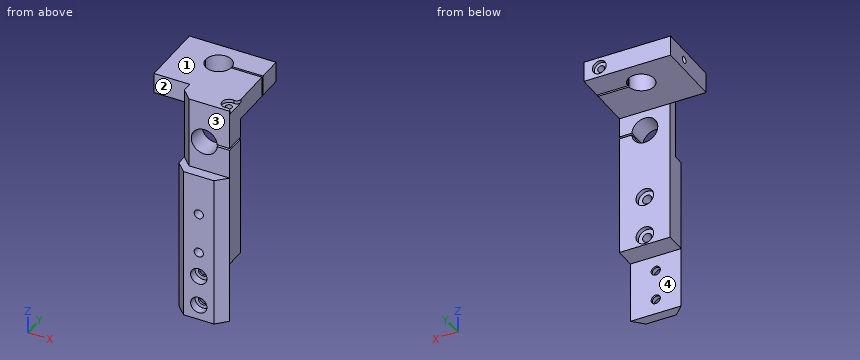
from build123d import *

# Parameters (mm, degrees)
SKETCH1_W                       = 24.85
SKETCH1_H                       = 110
BOSS_EXTRUDE1_DEPTH             = 15
SKETCH2_W                       = 24.85
SKETCH2_H                       = 30
CUT_EXTRUDE1_DEPTH              = 10
SKETCH4_W                       = 35
SKETCH4_H                       = 5
CUT_EXTRUDE3_DEPTH              = 63.189408262
SKETCH5_W                       = 17.575
SKETCH5_H                       = 10
BOSS_EXTRUDE2_DEPTH             = 10
SKETCH6_W                       = 42.425
SKETCH6_H                       = 10
BOSS_EXTRUDE3_DEPTH             = 32.42
CHAMFER2_SIZE                   = 5
SKETCH7_R                       = 6.375
CUT_EXTRUDE4_DEPTH              = 71.541168122
SKETCH8_R                       = 6.375
CUT_EXTRUDE5_DEPTH              = 115.667590888
CBORE_FOR_M4_SHCS1_D            = 4.5
CBORE_FOR_M4_SHCS1_DEPTH        = 10.1
CBORE_FOR_M4_SHCS1_CBORE_D      = 8
CBORE_FOR_M4_SHCS1_CBORE_DEPTH  = 4
CBORE_FOR_M4_SHCS1_TIP          = 1.351936393
M4X0_7_TAPPED_HOLE1_D           = 3.3
SKETCH15_W                      = 17.575
SKETCH15_H                      = 10
CUT_EXTRUDE6_DEPTH              = 115.667590888
CHAMFER6_SIZE                   = 5
SKETCH16_W                      = 15
SKETCH16_H                      = 1
CUT_EXTRUDE7_DEPTH              = 71.541168122
CBORE_FOR_M3_SBHCS1_D           = 3.2
CBORE_FOR_M3_SBHCS1_DEPTH       = 19.5
CBORE_FOR_M3_SBHCS1_CBORE_D     = 6.7
CBORE_FOR_M3_SBHCS1_CBORE_DEPTH = 1.65
M3X0_5_TAPPED_HOLE1_D           = 2.5
M3X0_5_TAPPED_HOLE1_DEPTH       = 7.5
M3X0_5_TAPPED_HOLE1_TIP         = 0.751075774
CUT_EXTRUDE8_REACH              = 125.485
SKETCH24_W                      = 22
SKETCH24_H                      = 1
CBORE_FOR_M3_SBHCS2_D           = 3.4
CBORE_FOR_M3_SBHCS2_DEPTH       = 11.92
CBORE_FOR_M3_SBHCS2_CBORE_D     = 6.7
CBORE_FOR_M3_SBHCS2_CBORE_DEPTH = 1.65
M3X0_5_TAPPED_HOLE2_D           = 2.5
M3X0_5_TAPPED_HOLE2_DEPTH       = 7.5
M3X0_5_TAPPED_HOLE2_TIP         = 0.751075774
M4X0_7_TAPPED_HOLE2_D           = 3.3
M4X0_7_TAPPED_HOLE2_DEPTH       = 10.1
M4X0_7_TAPPED_HOLE2_TIP         = 0.991420021
CBORE_FOR_M4_SBHCS1_D           = 4.5
CBORE_FOR_M4_SBHCS1_CBORE_D     = 8.6
CBORE_FOR_M4_SBHCS1_CBORE_DEPTH = 2.2
FILLET2_R                       = 2


with BuildPart() as part:
    # Sketch1 → Boss-Extrude1 (new body)
    with BuildSketch(Plane(origin=(0, 0, 0), x_dir=(1, 0, 0), z_dir=(0, 1, 0))):
        Rectangle(SKETCH1_W, SKETCH1_H)
    extrude(amount=BOSS_EXTRUDE1_DEPTH)

    # Sketch2 → Cut-Extrude1 (cut)
    with BuildSketch(Plane(origin=(0, 15, 0), x_dir=(1, 0, 0), z_dir=(0, 1, 0))):
        with Locations((0, 40)):
            Rectangle(SKETCH2_W, SKETCH2_H)
    extrude(amount=-CUT_EXTRUDE1_DEPTH, mode=Mode.SUBTRACT)

    # Sketch4 → Cut-Extrude3 (cut, through all)
    with BuildSketch(Plane.ZY.offset(12.425)):
        with Locations((37.5, 2.5)):
            Rectangle(SKETCH4_W, SKETCH4_H)
    extrude(amount=-CUT_EXTRUDE3_DEPTH, mode=Mode.SUBTRACT)

    # Sketch5 → Boss-Extrude2 (add)
    with BuildSketch(Plane(origin=(0, 15, 0), x_dir=(1, 0, 0), z_dir=(0, 1, 0))):
        with Locations((-21.2125, -50)):
            Rectangle(SKETCH5_W, SKETCH5_H)
    extrude(amount=-BOSS_EXTRUDE2_DEPTH)

    # Sketch6 → Boss-Extrude3 (add)
    with BuildSketch(Plane(origin=(0, 15, 0), x_dir=(1, 0, 0), z_dir=(0, 1, 0))):
        with Locations((-8.7875, -50)):
            Rectangle(SKETCH6_W, SKETCH6_H)
    extrude(amount=BOSS_EXTRUDE3_DEPTH)

    # Chamfer2
    chamfer2_edges = [part.edges().sort_by_distance(p)[0] for p in [
        (12.425, 0, -17.5),
        (-12.425, 0, -17.5),
    ]]
    chamfer(chamfer2_edges, length=CHAMFER2_SIZE)

    # Sketch7 → Cut-Extrude4 (cut, through all)
    with BuildSketch(Plane(origin=(0, 15, 0), x_dir=(1, 0, 0), z_dir=(0, 1, 0))):
        with Locations(Location((0, -35, 0), (0, 0, 270))):
            Circle(SKETCH7_R)
    extrude(amount=-CUT_EXTRUDE4_DEPTH, mode=Mode.SUBTRACT)

    # Sketch8 → Cut-Extrude5 (cut, through all)
    with BuildSketch(Plane(origin=(0, 0, 45), x_dir=(-1, 0, 0), z_dir=(0, 0, -1))):
        with Locations((9, 35)):
            Circle(SKETCH8_R)
    extrude(amount=-CUT_EXTRUDE5_DEPTH, mode=Mode.SUBTRACT)

    # CBORE for M4 SHCS1
    with Locations(Plane(origin=(0, 0, 0), x_dir=(-1, 0, 0), z_dir=(0, -1, 0))):
        with Locations((0, 47.5), (0, 32.5)):
            CounterBoreHole(CBORE_FOR_M4_SHCS1_D / 2, CBORE_FOR_M4_SHCS1_CBORE_D / 2, CBORE_FOR_M4_SHCS1_CBORE_DEPTH, depth=CBORE_FOR_M4_SHCS1_DEPTH)
            with Locations((0, 0, -(CBORE_FOR_M4_SHCS1_DEPTH + CBORE_FOR_M4_SHCS1_TIP / 2))):  # 118° drill point
                Cone(0, CBORE_FOR_M4_SHCS1_D / 2, CBORE_FOR_M4_SHCS1_TIP, mode=Mode.SUBTRACT)

    # M4x0.7 Tapped Hole1 (through all)
    with Locations(Plane(origin=(0, 0, 0), x_dir=(-1, 0, 0), z_dir=(0, -1, 0))):
        with Locations((0, 20), (0, 0)):
            Hole(M4X0_7_TAPPED_HOLE1_D / 2)

    # Sketch15 → Cut-Extrude6 (cut, through all)
    with BuildSketch(Plane(origin=(0, 0, 45), x_dir=(-1, 0, 0), z_dir=(0, 0, -1))):
        with Locations((21.2125, 10)):
            Rectangle(SKETCH15_W, SKETCH15_H)
    extrude(amount=-CUT_EXTRUDE6_DEPTH, mode=Mode.SUBTRACT)

    # Chamfer6
    chamfer6_edges = [part.edges().sort_by_distance(p)[0] for p in [
        (-12.425, 5, 37.5),
    ]]
    chamfer(chamfer6_edges, length=CHAMFER6_SIZE)

    # Sketch16 → Cut-Extrude7 (cut, through all)
    with BuildSketch(Plane(origin=(0, 15, 0), x_dir=(1, 0, 0), z_dir=(0, 1, 0))):
        with Locations((12.425, -35)):
            Rectangle(SKETCH16_W, SKETCH16_H)
    extrude(amount=-CUT_EXTRUDE7_DEPTH, mode=Mode.SUBTRACT)

    # CBORE for M3 SBHCS1
    with Locations(Plane(origin=(9.390180955, 10, 55), x_dir=(1, 0, 0), z_dir=(0, 0, 1))):
        with Locations((0, 0)):
            CounterBoreHole(CBORE_FOR_M3_SBHCS1_D / 2, CBORE_FOR_M3_SBHCS1_CBORE_D / 2, CBORE_FOR_M3_SBHCS1_CBORE_DEPTH, depth=CBORE_FOR_M3_SBHCS1_DEPTH)

    # M3x0.5 Tapped Hole1
    with Locations(Plane.XY.offset(34.5)):
        with Locations((9.390180955, 10)):
            Hole(M3X0_5_TAPPED_HOLE1_D / 2, depth=M3X0_5_TAPPED_HOLE1_DEPTH)
            with Locations((0, 0, -(M3X0_5_TAPPED_HOLE1_DEPTH + M3X0_5_TAPPED_HOLE1_TIP / 2))):  # 118° drill point
                Cone(0, M3X0_5_TAPPED_HOLE1_D / 2, M3X0_5_TAPPED_HOLE1_TIP, mode=Mode.SUBTRACT)

    # Sketch24 → Cut-Extrude8 (cut, up to next)
    with BuildSketch(Plane.XY.offset(55), mode=Mode.PRIVATE) as cut_extrude8_sk1:
        with Locations((1.425, 35)):
            Rectangle(SKETCH24_W, SKETCH24_H)
    cut_extrude8_tool1 = extrude(cut_extrude8_sk1.sketch, amount=-CUT_EXTRUDE8_REACH, mode=Mode.PRIVATE) & part.part
    add(cut_extrude8_tool1.solids().sort_by_distance((1.425, 35, 55))[0], mode=Mode.SUBTRACT)

    # CBORE for M3 SBHCS2
    with Locations(Plane(origin=(0, 47.42, 0), x_dir=(1, 0, 0), z_dir=(0, 1, 0))):
        with Locations((4.890180955, -50)):
            CounterBoreHole(CBORE_FOR_M3_SBHCS2_D / 2, CBORE_FOR_M3_SBHCS2_CBORE_D / 2, CBORE_FOR_M3_SBHCS2_CBORE_DEPTH, depth=CBORE_FOR_M3_SBHCS2_DEPTH)

    # M3x0.5 Tapped Hole2
    with Locations(Plane(origin=(0, 34.5, 0), x_dir=(1, 0, 0), z_dir=(0, 1, 0))):
        with Locations((4.890180955, -50)):
            Hole(M3X0_5_TAPPED_HOLE2_D / 2, depth=M3X0_5_TAPPED_HOLE2_DEPTH)
            with Locations((0, 0, -(M3X0_5_TAPPED_HOLE2_DEPTH + M3X0_5_TAPPED_HOLE2_TIP / 2))):  # 118° drill point
                Cone(0, M3X0_5_TAPPED_HOLE2_D / 2, M3X0_5_TAPPED_HOLE2_TIP, mode=Mode.SUBTRACT)

    # M4x0.7 Tapped Hole2
    with Locations(Plane.ZY.offset(30)):
        with Locations((50, 35)):
            Hole(M4X0_7_TAPPED_HOLE2_D / 2, depth=M4X0_7_TAPPED_HOLE2_DEPTH)
            with Locations((0, 0, -(M4X0_7_TAPPED_HOLE2_DEPTH + M4X0_7_TAPPED_HOLE2_TIP / 2))):  # 118° drill point
                Cone(0, M4X0_7_TAPPED_HOLE2_D / 2, M4X0_7_TAPPED_HOLE2_TIP, mode=Mode.SUBTRACT)

    # CBORE for M4 SBHCS1 (through all)
    with Locations(Plane(origin=(0, 15, 0), x_dir=(1, 0, 0), z_dir=(0, 1, 0))):
        with Locations((0, 20), (0, 0)):
            CounterBoreHole(CBORE_FOR_M4_SBHCS1_D / 2, CBORE_FOR_M4_SBHCS1_CBORE_D / 2, CBORE_FOR_M4_SBHCS1_CBORE_DEPTH)

    # Fillet2
    # the kernel refuses this fillet: 2 mm, written as the material it takes off along each edge
    with BuildSketch(Plane(origin=(12.425, 11.418581462, 53.35), x_dir=(0, 1, 0), z_dir=(0, 0, 1))) as fillet2_piece_1:
        with BuildLine():
            CenterArc((3.83038506, 2), FILLET2_R, 168.847320213, 101.152679787)
            Line((1.868154584, 2.386848241), (1.828909975, 2.394585206))
            ThreePointArc((1.828909975, 2.394585206), (1.187961295, 0.994712466), (-0.016938286, 0.036236645))
            Line((-0.016938286, 0.036236645), (0, -0.04))
            Line((0, -0.04), (3.83038506, -0.04))
            Line((3.83038506, -0.04), (3.83038506, 0))
        make_face()
    extrude(amount=11.225962649, mode=Mode.SUBTRACT)
    with BuildSketch(Plane(origin=(12.425, 8.581418538, 53.35), x_dir=(0, -1, 0), z_dir=(0, 0, 1))) as fillet2_piece_2:
        with BuildLine():
            CenterArc((3.827369434, -1.984819427), FILLET2_R, 97.063855439, 94.254577376)
            Line((1.866266295, -2.377342649), (1.827044233, -2.385193113))
            ThreePointArc((1.827044233, -2.385193113), (1.18500762, -0.99094432), (-0.016938286, -0.036236645))
            Line((-0.016938286, -0.036236645), (0, 0.04))
            ThreePointArc((0, 0.04), (1.790709269, 0.04), (3.57649952, 0.039696389))
            Line((3.57649952, 0.039696389), (3.581418538, 0))
        make_face()
    extrude(amount=10.603546345, mode=Mode.SUBTRACT)


solid = part.part
The listing builds one solid part. Answer for the finished solid, in the listing's coordinates (mm). Face numbers are marked on the shaded views. A direction names the side the tool comes from. Round coordinates to 2 decimals unless told otherwise and drop trailing zeros. Write each loop counter-clockwise with the first axis right and the second up, starting at its lowest first coordinate (ties: lowest second). Pieces come first, ordered by that corner, then holes. Notation, with made-up numbers: M -15,35 L 8,35 A20 cw 8,65 Z; hole C -13,34 d7. An arc over 180 degrees is marked long. Write each question's results on one line, items separated by ' | '. Start each with the question number.
Item 1: A cutting plane is placed at D-D on y = 22. Write down the section's boundary in (x, z) (3 decimals).
Item 2: Flat-ended cylindrical pins translate along their axes: pin 1 Ø6 at (x, z) = (0, -32.5) entering from +Y; pin 2 Ø4 at (x, y) = (-18, 14.5) entering from -Z; pin 3 Ø1 at (x, z) = (-7.5, 12) entering from +Y. Find the tip coordinate at first contact, or state that the pin passes through.
Item 3: Straight lines are drawn through the part: L1, parallel to Z at x = 0, y = 1.25; L2, parallel to Z at x = 0, y = 4.65; L3, parallel to Y at x = 3, z = -21.5. For each, find the intervals that lie inside material, in ascending order. Write a range as [from, to].
Item 4: A cutting plane is placed at A-A on z = 37.5. Write down the section's boundary in (x, y) (3 decimals), and give its area (3 significant figures).
Item 5: A cutting plane is placed at C-C on z = -20. Write down the section's boundary in (x, y) (3 decimals), and give its area (3 significant figures).
Item 6: A cutting plane is placed at B-B on x = -23. Write down the section's boundary in (y, z).
Item 7: For the marked faces 1, 2, 3 and 4, determine the directions among +Z, -Z, +X, -X, +Y, -Y from which every point of the face is accessible in a straight line to the end or side of a thin tool.
Check sheet entries:
1) outline: M -30,45 L 12.425,45 L 12.425,55 L -30,55 Z
2) pin 1: y = 5 | pin 2: z = 45 | pin 3: y = 15
3) L1: [-55, -51.5], [-43.5, -36.5], [-28.5, -22.25], [-17.75, -2.25], [2.25, 20] | L2: [-55, -49.75], [-45.25, -34.75], [-30.25, -22.25], [-17.75, -2.25], [2.25, 20] | L3: [0, 12.8]
4) outline: M -12.425,10 L -7.425,5 L -5.864,5 L -5.864,15 L -12.425,15 Z; M 5.864,5 L 12.425,5 L 12.425,15 L 5.864,15 Z; hole C 9.39,10 d3.2 | area: 111 mm²
5) outline: M -12.425,5 L -7.425,0 L -2.25,0 L -2.25,12.8 L -4.3,12.8 L -4.3,15 L -12.425,15 Z; M 2.25,0 L 7.425,0 L 12.425,5 L 12.425,15 L 4.3,15 L 4.3,12.8 L 2.25,12.8 Z | area: 271 mm²
6) outline: M 15,45 L 47.42,45 L 47.42,55 L 15,55 Z; hole C 35,50 d3.3
7) face 1: +Z, +X, -X, +Y, -Y | face 2: +Z, -Z, -X, -Y | face 3: +Z, +X, -X, -Y | face 4: -Z, +X, -X, +Y
